The listing builds one solid part. Answer for the finished solid, in the listing's coordinates (mm). Face numbers are marked on the shaded views. A direction names the side the tool comes from. Give positions to 0.01 mm unless a question says otherwise; leave off trailing zeros. Order: outer loops, then holes, each group sorted by start corner. A loop starts at its lowest first (then second) coordinate and runs counter-clockwise, first axis right, second up. Notation, with made-up numbers: (26.25, 69.5) -> (80.25, 69.5) arc R21 cw to (80.25, 98.5) -> close; hole circle Ø5 at (31.5, 23). An arc over 180 degrees is marked (long way). Answer as a JSON object with one key per item and string values. Group by question number.
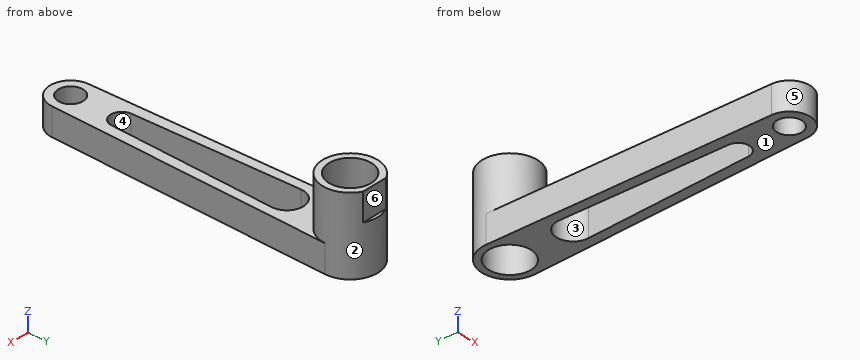
```python
from build123d import *

# Parameters (mm, degrees)
SKETCH1_R           = 4.515
BOSS_EXTRUDE2_DEPTH = 10
SKETCH1_6_R         = 10
SKETCH1_6_R_2       = 7.675
BOSS_EXTRUDE3_DEPTH = 27.94
SKETCH2_W           = 20.025396677
SKETCH2_H           = 9.808205023
CUT_EXTRUDE1_DEPTH  = 10


with BuildPart() as part:
    # Sketch1 → Boss-Extrude2 (new body)
    with BuildSketch(Plane.XY):
        with BuildLine():
            Line((-9.996972195, -0.246062876), (-7.497729139, -101.784547426))
            ThreePointArc((-7.497729139, -101.784547426), (1.58e-07, -109.1), (7.497729147, -101.784547111))
            Line((7.497729147, -101.784547111), (9.996972197, -0.246062766))
            ThreePointArc((9.996972197, -0.246062766), (5.5e-08, -10), (-9.996972195, -0.246062876))
        make_face()
        with BuildLine():
            ThreePointArc((-5.996665745, -23.199999845), (2.1e-08, -17), (5.996665744, -23.199999888))
            Line((5.996665744, -23.199999888), (3.997777167, -83.133333141))
            ThreePointArc((3.997777167, -83.133333141), (1.93e-07, -87), (-3.997777154, -83.133333527))
            Line((-3.997777154, -83.133333527), (-5.996665745, -23.199999845))
        make_face(mode=Mode.SUBTRACT)
        with Locations((0, -101.6)):
            Circle(SKETCH1_R, mode=Mode.SUBTRACT)
    extrude(amount=BOSS_EXTRUDE2_DEPTH)

    # Sketch1_6 → Boss-Extrude3 (add)
    with BuildSketch(Plane.XY):
        with Locations(Location((0, 0, 0), (0, 0, 181.409979402))):
            Circle(SKETCH1_6_R)
        Circle(SKETCH1_6_R_2, mode=Mode.SUBTRACT)
    extrude(amount=BOSS_EXTRUDE3_DEPTH)

    # Sketch2 → Cut-Extrude1 (cut)
    with BuildSketch(Plane.XY.offset(27.94)):
        with Locations((-0.020605473, 13.754102512)):
            Rectangle(SKETCH2_W, SKETCH2_H)
    extrude(amount=-CUT_EXTRUDE1_DEPTH, mode=Mode.SUBTRACT)


solid = part.part
```
(1) A cutting plane is placed at B-B (y = -57.5). Determine the outline of the cut face in (x, z).
(2) For a pull along X with two mould halves and no side action, classify the marked faces 4, 5 and 6 as +X half, -X half, draft (parallel to the pull), parting line (faces both ways), or undercut.
(3) Which of the six approach directions +Z, -Z, +X, -X, +Y, -Y give full straight-line access (tool end or side, diameter ignored) to the marked faces 1, 2 and 3?
(4) Flat-ended cylindrical pins translate along their axes: pin 1 Ø1.5 at (x, y) = (8, -43) entering from +Z; pin 2 Ø1.5 at (x, z) = (1, 6.5) entering from +Y; pin 3 Ø0.6 at (x, y) = (2.5, 9.5) entering from +Z. Find the tip coordinate at first contact, or state that the pin passes through.
(5) A cutting plane is placed at C-C (z = 21.25). Determine the outline of the cut face in (x, y) (3 decimals).
(6) A cutting plane is placed at A-A (x = 0). Determine the outline of the cut face in (y, z) (3 decimals).
(7) Find the intervals of material crossed by line 1 along Y through (x, z) = (0, 16.75) (3 decimals); line 2 along Y through (x, z) = (5, 11.25); line 3 along Z through (x, y) = (8, -58), in increasing order. Write a range as [from, to].
(8) A cutting plane is placed at D-D (y = -36). Determine the outline of the cut face in (x, z), and give its area (3 significant figures).
Check sheet entries:
{
 "1": {"outline": "(-8.59, 0) -> (-4.85, 0) -> (-4.85, 10) -> (-8.59, 10) -> close; (4.85, 0) -> (8.59, 0) -> (8.59, 10) -> (4.85, 10) -> close"},
 "2": {"face 4": "undercut", "face 5": "parting line", "face 6": "draft"},
 "3": {"face 1": "-Z, +X, -X, +Y, -Y", "face 2": "+Z", "face 3": "+Z, -Z"},
 "4": {"pin 1": "stops at z = 10", "pin 2": "stops at y = 10", "pin 3": "stops at z = 17.94"},
 "5": {"outline": "(-4.656, 8.85) arc R10 ccw (long way) to (4.656, 8.85) -> close; hole circle Ø15.35 at (0, 0)"},
 "6": {"outline": "(-109.1, 0) -> (-106.115, 0) -> (-106.115, 10) -> (-109.1, 10) -> close; (-97.085, 0) -> (-87, 0) -> (-87, 10) -> (-97.085, 10) -> close; (-17, 0) -> (-7.675, 0) -> (-7.675, 27.94) -> (-10, 27.94) -> (-10, 10) -> (-17, 10) -> close; (7.675, 0) -> (10, 0) -> (10, 17.94) -> (8.85, 17.94) -> (8.85, 27.94) -> (7.675, 27.94) -> close"},
 "7": {"line 1": "y = [-10, -7.675], [7.675, 10]", "line 2": "y = [-8.66, -5.82], [5.82, 8.66]", "line 3": "z = [0, 10]"},
 "8": {"outline": "(-9.12, 0) -> (-5.57, 0) -> (-5.57, 10) -> (-9.12, 10) -> close; (5.57, 0) -> (9.12, 0) -> (9.12, 10) -> (5.57, 10) -> close", "area": "70.9 mm2"}
}
